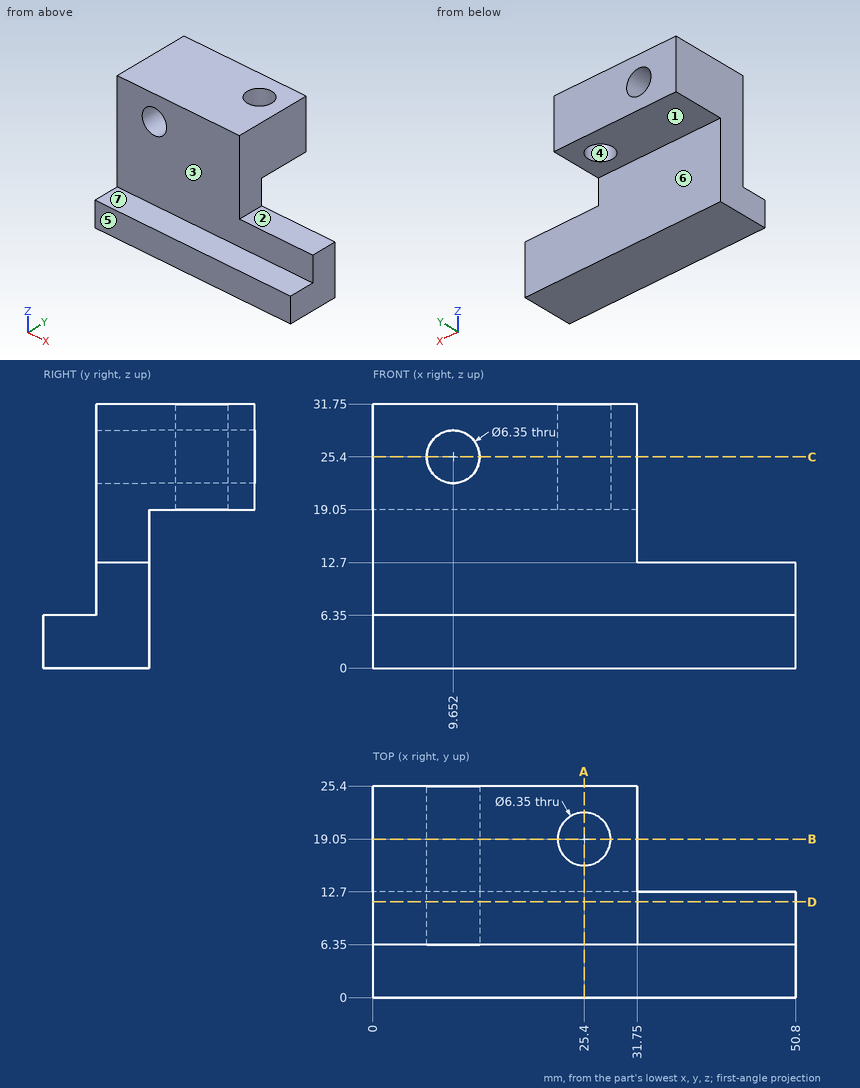
Geometry: see drawing. Coordinates: mm, zero at the bounding-box minimum. A direction names the side the tool comes from. Coordinates: 2 decimals unless noted, no trailing zeros. Loops run counter-clockwise (first coordinate to the right, second up) from the corner with the lowest first, then second, coordinate; pieces in that order, holes last.
(1) Section A-A on x = 25.4. Return the cut outline in (y, z) (3 decimals), then the cut area to 3 significant figures.
(2) Section D-D on y = 11.5. Return the cut outline in (x, z) (3 decimals).
(3) Section C-C on z = 25.4. Return the cut outline in (x, y) (3 decimals).
(4) Section B-B on y = 19.05. Return the cut outline in (x, z) (3 decimals).
(5) Set-up query: the marked faces 1, 2 and 3. Return all of +Z, -Z, +X, -X, +Y, -Y with unobstructed straight access to the full face (end or side cutting, diameter ignored); none if empty.
(6) First-contact query: pin 1 Ø7 at (x, y) = (45, 9.5) entering from +Z; pin 2 Ø5 at (x, y) = (25.4, 19.05) entering from +Z; pin 3 Ø1 at (x, z) = (19, 5.5) entering from +Y; pin 4 Ø6.5 at (x, y) = (16, 20.5) entering from -Z. Flat tips, straight axial feed; report the tip coordinate or a pass-through.
(7) Material intervals for probe 1 along Y at (x, z) = (25.4, 23.75) (3 decimals); probe 2 along Z at (x, y) = (47, 12); probe 3 along Z at (x, y) = (20, 4), sorted ascending.
(8) Pull-direction query (Y, two-part tool) for the marked faces 4, 5, 6 and 7; classes: released by +Y, released by -Y, zero draft, split by the parting line, or undercut.
Data:
1. outline: (0, 0) - (12.7, 0) - (12.7, 19.05) - (15.875, 19.05) - (15.875, 31.75) - (6.35, 31.75) - (6.35, 6.35) - (0, 6.35) - close; (22.225, 19.05) - (25.4, 19.05) - (25.4, 31.75) - (22.225, 31.75) - close
1. area: 323 mm2
2. outline: (0, 0) - (50.8, 0) - (50.8, 12.7) - (31.75, 12.7) - (31.75, 31.75) - (0, 31.75) - close; hole circle Ø6.35 at (9.652, 25.4)
3. outline: (0, 6.35) - (6.477, 6.35) - (6.477, 25.4) - (0, 25.4) - close; (12.827, 6.35) - (31.75, 6.35) - (31.75, 25.4) - (12.827, 25.4) - close; hole circle Ø6.35 at (25.4, 19.05)
4. outline: (0, 19.05) - (22.225, 19.05) - (22.225, 31.75) - (0, 31.75) - close; (28.575, 19.05) - (31.75, 19.05) - (31.75, 31.75) - (28.575, 31.75) - close; hole circle Ø6.35 at (9.652, 25.4)
5. face 1: -Z, +X, -X, +Y
5. face 2: +Z, +X, +Y, -Y
5. face 3: +Z, +X, -X, -Y
6. pin 1: stops at z = 12.7
6. pin 2: passes through
6. pin 3: stops at y = 12.7
6. pin 4: stops at z = 19.05
7. probe 1: y = 6.35 to 15.875, 22.225 to 25.4
7. probe 2: z = 0 to 12.7
7. probe 3: z = 0 to 6.35
8. face 4: undercut
8. face 5: released by -Y
8. face 6: released by +Y
8. face 7: zero draft
